Work out the finished part from the listing and answer in its coordinate system (mm). Face numbers are marked on the shaded views. A direction names the side the tool comes from. Coordinates: 2 decimals unless noted, no trailing zeros. Order: outer loops, then holes, each group sorted by start corner. A loop starts at its lowest first (then second) coordinate and runs counter-clockwise, first axis right, second up. Notation, with made-up numbers: (75, 74) - (101, 74) arc R19 ccw to (101, 83) - close; hole circle Ø6 at (71.5, 10). An arc over 180 degrees is marked (long way). Answer as a JSON object with one key per item and string values. Group by question number.
1) Section D-D (x = -2.75) is taken. Give the vertices of the cut face in (y, z), plus the area to 3 significant figures.
2) The mould has two halves that part along Y. Classify the marked faces 4 and 5: released by +Y, released by -Y, zero draft, split by the parting line, or undercut.
3) Section B-B (z = -21.95) is taken. Give the vertices of the cut face in (x, y) (3 decimals), plus the area to 3 significant figures.
4) A tool of negligible diameter and unlimited length cuts with its end or side. For the marked faces 1, 2 and 3, from which of +Z, -Z, +X, -X, +Y, -Y can it reach the whole face along a straight path? Write none if from no direction.
5) Each of these flat-tipped pins is pushed along its axis until it touches: P1, Ø4, axis at y = 0, z = 21.5, coming from the +X side; P2, Ø10, axis at x = 1, z = -9, coming from the +Y side; P3, Ø18, axis at y = -8, z = 8.5, coming from the -X side. Where does it stop, or does it pass through?
6) Section C-C (z = 0) is taken. Give the vertices of the cut face in (x, y), plus the area to 3 significant figures.
7) Find the intervals of material crossed by line 1 along X through (y, z) = (11.5, 3); line 2 along X through (y, z) = (-2, 23.5); line 3 along Y through (x, z) = (1.55, -21.95) (3 decimals), in increasing order.
8) Section A-A (y = 0) is taken. Count the separate pieces of the cut face and the enclosed holes in it, plus the area to 3 significant figures.
from build123d import *

# Parameters (mm, degrees)
ESQUISSE2_R             = 18.25
BOSS_EXTRU_1_DEPTH      = 5.25
ESQUISSE3_R             = 17.25
BOSS_EXTRU_2_DEPTH      = 2
ESQUISSE4_R             = 18.25
BOSS_EXTRU_3_DEPTH      = 5.25
ESQUISSE6_R             = 1.5
BOSS_EXTRU_4_DEPTH      = 2
ESQUISSE7_R             = 8
BOSS_EXTRU_5_DEPTH      = 2
ESQUISSE8_R             = 2.5
BOSS_EXTRU_6_DEPTH      = 10.5
CHANFREIN1_SIZE         = 0.25
ESQUISSE9_W             = 5
ESQUISSE9_H             = 1
ENL_V_MAT_EXTRU_1_DEPTH = 5


with BuildPart() as part:
    # Esquisse2 → Boss.-Extru.1 (new body)
    with BuildSketch(Plane(origin=(0, 0, 0), x_dir=(0, 0, -1), z_dir=(1, 0, 0))):
        with Locations(Location((0, 0, 0), (0, 0, 180))):
            Circle(ESQUISSE2_R)
    extrude(amount=BOSS_EXTRU_1_DEPTH)

    # Esquisse3 → Boss.-Extru.2 (add)
    with BuildSketch(Plane(origin=(5.25, 0, 0), x_dir=(0, 0, -1), z_dir=(1, 0, 0))):
        Circle(ESQUISSE3_R)
    extrude(amount=BOSS_EXTRU_2_DEPTH)

    # Esquisse4 → Boss.-Extru.3 (add)
    with BuildSketch(Plane(origin=(7.25, 0, 0), x_dir=(0, 0, -1), z_dir=(1, 0, 0))):
        with Locations(Location((0, 0, 0), (0, 0, 180))):
            Circle(ESQUISSE4_R)
    extrude(amount=BOSS_EXTRU_3_DEPTH)

    # Esquisse6 → Boss.-Extru.4 (add)
    # profile 1 of 2: a face of its own
    with BuildSketch(Plane.ZY):
        with BuildLine():
            ThreePointArc((23.313667029, -3.27763821), (25.5, 0), (23.313667029, 3.27763821))
            Line((23.313667029, 3.27763821), (17.312357631, 5.774493333))
            ThreePointArc((17.312357631, 5.774493333), (18.014064322, 2.925061814), (18.25, 0))
            ThreePointArc((18.25, 0), (18.014064322, -2.925061814), (17.312357631, -5.774493333))
            Line((17.312357631, -5.774493333), (23.313667029, -3.27763821))
        make_face()
        with Locations((21.95, 0)):
            Circle(ESQUISSE6_R, mode=Mode.SUBTRACT)
    # profile 2 of 2: a face of its own
    with BuildSketch(Plane.ZY):
        with BuildLine():
            ThreePointArc((-17.312357631, -5.774493333), (-18.25, 0), (-17.312357631, 5.774493333))
            Line((-17.312357631, 5.774493333), (-23.313667029, 3.27763821))
            ThreePointArc((-23.313667029, 3.27763821), (-25.5, 0), (-23.313667029, -3.27763821))
            Line((-23.313667029, -3.27763821), (-17.312357631, -5.774493333))
        make_face()
        with Locations((-21.95, 0)):
            Circle(ESQUISSE6_R, mode=Mode.SUBTRACT)
    extrude(amount=-BOSS_EXTRU_4_DEPTH)

    # Esquisse7 → Boss.-Extru.5 (add)
    with BuildSketch(Plane.ZY):
        Circle(ESQUISSE7_R)
    extrude(amount=BOSS_EXTRU_5_DEPTH)

    # Esquisse8 → Boss.-Extru.6 (add)
    with BuildSketch(Plane.ZY):
        with Locations(Location((0, 0, 0), (0, 0, 180))):
            Circle(ESQUISSE8_R)
    extrude(amount=BOSS_EXTRU_6_DEPTH)

    # Chanfrein1
    chanfrein1_edges = [part.edges().sort_by_distance(p)[0] for p in [
        (-10.5, 0, 2.5),
    ]]
    chamfer(chanfrein1_edges, length=CHANFREIN1_SIZE)

    # Esquisse9 → Enlèv. mat.-Extru.1 (cut)
    with BuildSketch(Plane.ZY.offset(10.5)):
        with Locations((0, 2.5)):
            Rectangle(ESQUISSE9_W, ESQUISSE9_H)
    extrude(amount=-ENL_V_MAT_EXTRU_1_DEPTH, mode=Mode.SUBTRACT)


solid = part.part
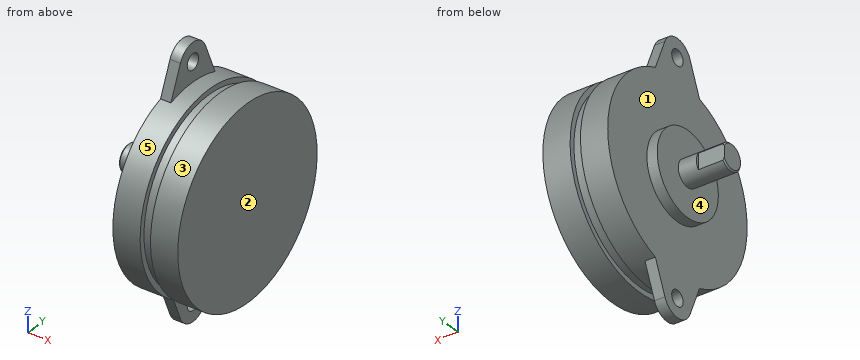
Report:
{
 "1": {"outline": "circle Ø5 at (0, 0)", "area": "19.6 mm²"},
 "2": {"face 4": "zero draft", "face 5": "split by the parting line"},
 "3": {"outline": "(0, -3.845) - (2, -3.845) - (2, -1.5) - (0, -1.5) - close; (0, 1.5) - (2, 1.5) - (2, 3.845) - (0, 3.845) - close", "area": "9.38 mm²"},
 "4": {"face 1": "-X", "face 2": "+Z, -Z, +X, +Y, -Y", "face 3": "+X"},
 "5": {"P1": "stops at x = 2", "P2": "stops at y = 17.81", "P3": "stops at x = -2"},
 "6": {"outline": "(-10.5, -2.25) - (-10.25, -2.5) - (-2, -2.5) - (-2, -8) - (0, -8) - (0, -18.25) - (5.25, -18.25) - (5.25, -17.25) - (7.25, -17.25) - (7.25, -18.25) - (12.5, -18.25) - (12.5, 18.25) - (7.25, 18.25) - (7.25, 17.25) - (5.25, 17.25) - (5.25, 18.25) - (0, 18.25) - (0, 8) - (-2, 8) - (-2, 2.5) - (-5.5, 2.5) - (-5.5, 2) - (-10.5, 2) - close", "area": "524 mm²"},
 "7": {"line 1": "x = 0 to 12.5", "line 2": "x = 0 to 2", "line 3": "y = -3.845 to -1.5, 1.5 to 3.845"},
 "8": {"separate pieces": "3", "enclosed holes": "0", "area": "544 mm²"}
}
